Part print with two shaded views. Sizes in mm from the minimum x, y, z corner. Round coordinates to 2 decimals unless told otherwise and drop trailing zeros. Order: outer loops, then holes, each group sorted by start corner. A loop starts at its lowest first (then second) coordinate and runs counter-clockwise, first axis right, second up. Notation, with made-up numbers: (72.5, 53) -> (86.5, 53) arc R20 cw to (86.5, 65) -> close; hole circle Ø1 at (-31.75, -39). An arc over 180 degrees is marked (long way). Put each result on its own line as item: value. Start each with the question number.
Q1. Cut at B-B, the plane y = 30. List the corners of the cut face in (x, z), and give its area (3 significant figures).
Q2. Flat gauge pin, fed straight in: P1, Ø22.5, axis at x = 250, y = 30, coming from the -Z side. Where does the tip first touch, or does it go through?
Q3. Cut at C-C, the plane z = 5.5. List the corners of the cut face in (x, y).
Q4. Probe L1, parallel to Y at x = 150, z = 9.75; L2, parallel to X at y = 14, z = 2.75; L3, parallel to X at y = 28, z = 2. List the from-to ranges inside material, lowest first.
Q5. Cut at D-D, the plane x = 150. List the corners of the cut face in (y, z), and give its area (3 significant figures).
Q6. Cut at A-A, the plane x = 50. List the corners of the cut face in (y, z), and give its area (3 significant figures).
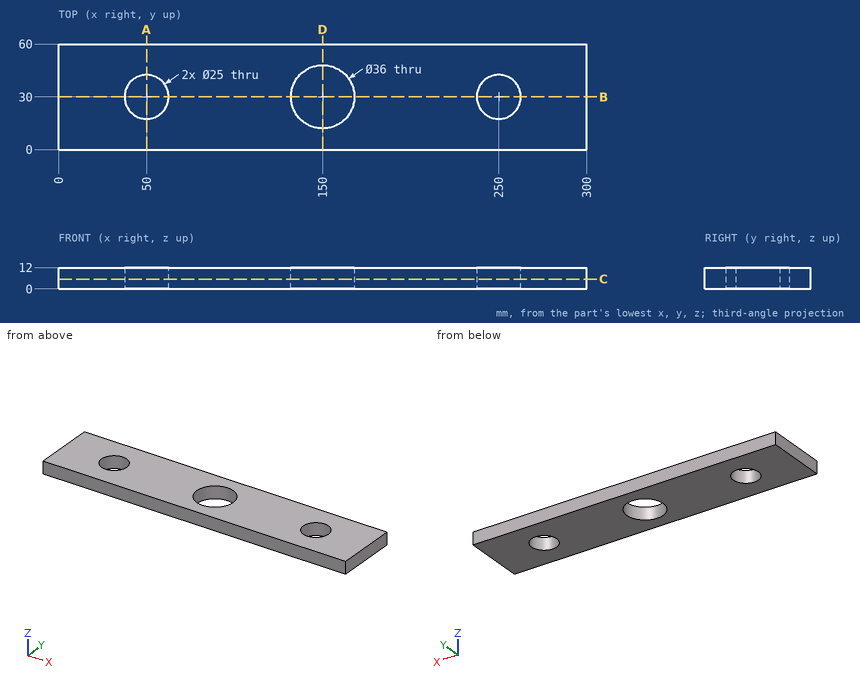
Ans:
1. outline: (0, 0) -> (37.5, 0) -> (37.5, 12) -> (0, 12) -> close; (62.5, 0) -> (132, 0) -> (132, 12) -> (62.5, 12) -> close; (168, 0) -> (237.5, 0) -> (237.5, 12) -> (168, 12) -> close; (262.5, 0) -> (300, 0) -> (300, 12) -> (262.5, 12) -> close
1. area: 2,570 mm^2
2. P1: passes through
3. outline: (0, 0) -> (300, 0) -> (300, 60) -> (0, 60) -> close; hole circle Ø25 at (50, 30); hole circle Ø36 at (150, 30); hole circle Ø25 at (250, 30)
4. L1: y = 0 to 12, 48 to 60
4. L2: x = 0 to 141.75, 158.25 to 300
4. L3: x = 0 to 37.66, 62.34 to 132.11, 167.89 to 237.66, 262.34 to 300
5. outline: (0, 0) -> (12, 0) -> (12, 12) -> (0, 12) -> close; (48, 0) -> (60, 0) -> (60, 12) -> (48, 12) -> close
5. area: 288 mm^2
6. outline: (0, 0) -> (17.5, 0) -> (17.5, 12) -> (0, 12) -> close; (42.5, 0) -> (60, 0) -> (60, 12) -> (42.5, 12) -> close
6. area: 420 mm^2
